Check sheet for the modelled part. Datum: model origin and axes. Units: mm. A direction names the side the tool comes from. Give positions to 0.01 mm unless a question says otherwise; leave off trailing zeros. Write each loop counter-clockwise with the first axis right and the second up, starting at its lowest first coordinate (ties: lowest second). Pieces come first, ordered by that corner, then holes. Notation, with made-up numbers: M 10,22 L 42,22 A21 cw 42,46 Z; hole C 69.25,-20.5 d10. An arc over 180 degrees is marked long. One line per item, written item: value. Start each with the question number.
from build123d import *

# Parameters (mm, degrees)
SKETCH1_W                 = 20.6
SKETCH1_H                 = 16
BOSS_EXTRUDE1_DEPTH       = 12.8
SKETCH2_W                 = 8.1
SKETCH2_H                 = 16
BOTTOM_CUT_DEPTH          = 1.1
FILL_PATTERN1_OUTLINE_W   = 8.1
FILL_PATTERN1_OUTLINE_H   = 16
FILL_PATTERN1_DEPTH       = 1.1
FILLET1_R                 = 2
SKETCH3_W                 = 8.1
SKETCH3_H                 = 14.8
TOP_CUT_DEPTH             = 7
M3X0_5_TAPPED_HOLE1_D     = 2.5
FILL_START                = 5.8
FILL_PATTERN2_OUTLINE_W   = 8.1
FILL_PATTERN2_OUTLINE_H   = 14.8
FILL_PATTERN2_DEPTH       = 7
FILL_START_2              = 1.1
FILL_PATTERN2_2_OUTLINE_R = 1.25
FILL_PATTERN2_2_DEPTH     = 4.7
SKETCH7_W                 = 1.5
SKETCH7_H                 = 4.4
BOSS_EXTRUDE2_DEPTH       = 4
CUT_EXTRUDE1_REACH        = 29.76
SKETCH8_R                 = 0.75
FILLET2_R                 = 0.5
LPATTERN1_COUNT           = 2
LPATTERN1_PITCH           = 10
FILLET2_OF_LPATTERN1_R    = 0.5
MIRROR1_START             = 8.8
MIRROR1_OUTLINE_R         = 0.75
MIRROR1_DEPTH             = 1.5


# Read off the part's stored shape, not the designer's step: Fill Pattern1, Fill Pattern2, Mirror1
with BuildPart() as part:
    # Sketch1 → Boss-Extrude1 (new body)
    with BuildSketch(Plane(origin=(0, 0, 0), x_dir=(1, 0, 0), z_dir=(0, 1, 0))):
        Rectangle(SKETCH1_W, SKETCH1_H)
    extrude(amount=BOSS_EXTRUDE1_DEPTH)

    # Sketch2 → BOTTOM CUT (cut)
    with BuildSketch(Plane.XZ):
        with Locations((-4.75, 0)):
            Rectangle(SKETCH2_W, SKETCH2_H)
    extrude(amount=-BOTTOM_CUT_DEPTH, mode=Mode.SUBTRACT)

    # Fill Pattern1 outline → Fill Pattern1 (cut)
    with BuildSketch(Plane(origin=(0, 0, 0), x_dir=(1, 0, 0), z_dir=(0, 1, 0))):
        with Locations((4.75, 0)):
            Rectangle(FILL_PATTERN1_OUTLINE_W, FILL_PATTERN1_OUTLINE_H)
    extrude(amount=FILL_PATTERN1_DEPTH, mode=Mode.SUBTRACT)

    # Fillet1
    fillet1_edges = [part.edges().sort_by_distance(p)[0] for p in [
        (0, 12.8, 8),
    ]]
    fillet(fillet1_edges, radius=FILLET1_R)

    # Sketch3 → TOP CUT (cut)
    with BuildSketch(Plane(origin=(0, 12.8, 0), x_dir=(1, 0, 0), z_dir=(0, 1, 0))):
        with Locations((-4.75, -0.6)):
            Rectangle(SKETCH3_W, SKETCH3_H)
    extrude(amount=-TOP_CUT_DEPTH, mode=Mode.SUBTRACT)

    # M3x0.5 Tapped Hole1 (through all)
    with Locations(Plane(origin=(0, 5.8, 0), x_dir=(1, 0, 0), z_dir=(0, 1, 0))):
        with Locations((-4.75, -1)):
            Hole(M3X0_5_TAPPED_HOLE1_D / 2)

    # Fill Pattern2 outline → Fill Pattern2 (cut)
    with BuildSketch(Plane(origin=(0, 0, 0), x_dir=(1, 0, 0), z_dir=(0, 1, 0)).offset(FILL_START)):
        with Locations((4.75, -0.6)):
            Rectangle(FILL_PATTERN2_OUTLINE_W, FILL_PATTERN2_OUTLINE_H)
    extrude(amount=FILL_PATTERN2_DEPTH, mode=Mode.SUBTRACT)

    # Fill Pattern2 2 outline → Fill Pattern2 2 (cut)
    with BuildSketch(Plane(origin=(0, 0, 0), x_dir=(1, 0, 0), z_dir=(0, 1, 0)).offset(FILL_START_2)):
        with Locations((4.75, -1)):
            Circle(FILL_PATTERN2_2_OUTLINE_R)
    extrude(amount=FILL_PATTERN2_2_DEPTH, mode=Mode.SUBTRACT)

    # Sketch7 → Boss-Extrude2 (add)
    with BuildSketch(Plane(origin=(0, 12.8, 0), x_dir=(1, 0, 0), z_dir=(0, 1, 0))):
        with Locations((-9.55, 5.8)):
            Rectangle(SKETCH7_W, SKETCH7_H)
    boss_extrude2 = extrude(amount=BOSS_EXTRUDE2_DEPTH)

    # Sketch8 → Cut-Extrude1 (cut, up to next)
    with BuildSketch(Plane.ZY.offset(10.3), mode=Mode.PRIVATE) as cut_extrude1_sk1:
        with Locations((-5.8, 14.8)):
            Circle(SKETCH8_R)
    cut_extrude1_tool1 = extrude(cut_extrude1_sk1.sketch, amount=-CUT_EXTRUDE1_REACH, mode=Mode.PRIVATE) & part.part
    cut_extrude1 = cut_extrude1_tool1.solids().sort_by_distance((-10.3, 14.8, -5.8))[0]
    add(cut_extrude1, mode=Mode.SUBTRACT)

    # Fillet2
    fillet2_edges = [part.edges().sort_by_distance(p)[0] for p in [
        (-9.55, 16.8, -3.6),
        (-9.55, 16.8, -8),
    ]]
    fillet(fillet2_edges, radius=FILLET2_R)

    # LPattern1: Boss-Extrude2, Cut-Extrude1 ×2
    with Locations(*[(0, 0, i * LPATTERN1_PITCH) for i in range(1, LPATTERN1_COUNT)]):
        add(boss_extrude2)
        add(cut_extrude1, mode=Mode.SUBTRACT)

    # Fillet2 of LPattern1
    fillet2_of_lpattern1_edges = [part.edges().sort_by_distance(p)[0] for p in [
        (-9.55, 16.8, 6.4),
        (-9.55, 16.8, 2),
    ]]
    fillet(fillet2_of_lpattern1_edges, radius=FILLET2_OF_LPATTERN1_R)

    # Mirror1 outline → Mirror1 (add)
    # profile 1 of 2: a face of its own
    with BuildSketch(Plane.YZ.offset(MIRROR1_START)):
        with BuildLine():
            ThreePointArc((16.8, -4.1), (16.653553391, -3.746446609), (16.3, -3.6))
            Line((16.3, -3.6), (12.8, -3.6))
            Line((12.8, -3.6), (12.8, -8))
            Line((12.8, -8), (16.3, -8))
            ThreePointArc((16.3, -8), (16.653553391, -7.853553391), (16.8, -7.5))
            Line((16.8, -7.5), (16.8, -4.1))
        make_face()
        with Locations((14.8, -5.8)):
            Circle(MIRROR1_OUTLINE_R, mode=Mode.SUBTRACT)
    # profile 2 of 2: a face of its own
    with BuildSketch(Plane.YZ.offset(MIRROR1_START)):
        with BuildLine():
            Line((12.8, 6.4), (12.8, 2))
            Line((12.8, 2), (16.3, 2))
            ThreePointArc((16.3, 2), (16.653553391, 2.146446609), (16.8, 2.5))
            Line((16.8, 2.5), (16.8, 5.9))
            ThreePointArc((16.8, 5.9), (16.653553391, 6.253553391), (16.3, 6.4))
            Line((16.3, 6.4), (12.8, 6.4))
        make_face()
        with Locations((14.8, 4.2)):
            Circle(MIRROR1_OUTLINE_R, mode=Mode.SUBTRACT)
    extrude(amount=MIRROR1_DEPTH)


solid = part.part
1) Cross-section at A-A (x = -4.75). Record the boundary of the cut face in (y, z).
2) Gauge pin test, flat ends, axial feed: pin 1 (6.5 mm diameter, centred on x = -4.5, z = 2.5, fed in from +Y); pin 2 (7 mm diameter, centred on x = 1, z = 2, fed in from +Y); pin 3 (0.8 mm diameter, centred on x = -10, y = 14.5, fed in from +Z). Record the tip position at first contact, or that the pin passes through.
3) Material ranges on L1, parallel to X at y = 11.5, z = 0; L2, parallel to Z at x = 4.75, y = 3.05; L3, parallel to Z at x = 9.9, y = 14.8, recorded low to high. Write a range as from..to.
4) Draft check along X on faces 1 (the flat face through (-8.8, 0.5, -0.1)), 2 (the flat face through (10, 12.8, -1)), 3 (the flat face through (-10.3, 8, 0)). Enter one of: released by +X, released by -X, zero draft, split by the parting line, or undercut.
5) Cross-section at B-B (y = 14.8). State how many separate pieces and enclosed holes the cut face has, plus the area to 3 significant figures.
6) Tool access check on faces 4 (the flat face through (8.8, 10, 0)), 5 (the flat face through (10, 15, -3.6)), 6 (the flat face through (0.7, 0.5, 0.1)), 7 (the flat face through (10, 15, 6.4)). Record the directions out of +Z, -Z, +X, -X, +Y, -Y that give a thin tool (end or side, any length) a straight path to the whole face; none if there is none.
7) Cross-section at D-D (y = 12.5). Record the boundary of the cut face in (x, z), plus the area to 3 significant figures.
8) Cross-section at C-C (z = 4.2). Record the boundary of the cut face in (x, y), plus the area to 3 significant figures.
Data:
1. outline: M 1.1,-8 L 12.8,-8 L 12.8,-6.8 L 5.8,-6.8 L 5.8,-0.25 L 1.1,-0.25 Z; M 1.1,2.25 L 5.8,2.25 L 5.8,8 L 1.1,8 Z
2. pin 1: stops at y = 5.8
2. pin 2: stops at y = 12.8
2. pin 3: stops at z = 6.4
3. L1: x = -10.3..-8.8, -0.7..0.7, 8.8..10.3
3. L2: z = -8..-0.25, 2.25..8
3. L3: z = -8..-6.55, -5.05..-3.6, 2..3.45, 4.95..6.4
4. face 1: undercut
4. face 2: zero draft
4. face 3: released by -X
5. separate pieces: 8
5. enclosed holes: 0
5. area: 17.4 mm2
6. face 4: +Z, +Y
6. face 5: +X, -X, +Y
6. face 6: +Z, -Z, -Y
6. face 7: +Z, +X, -X, +Y
7. outline: M -10.3,-8 L 10.3,-8 L 10.3,7.05 L 8.8,7.05 L 8.8,-6.8 L 0.7,-6.8 L 0.7,7.05 L -0.7,7.05 L -0.7,-6.8 L -8.8,-6.8 L -8.8,7.05 L -10.3,7.05 Z
7. area: 85.7 mm2
8. outline: M -10.3,0 L -8.8,0 L -8.8,1.1 L -0.7,1.1 L -0.7,0 L 0.7,0 L 0.7,1.1 L 8.8,1.1 L 8.8,0 L 10.3,0 L 10.3,14.05 L 8.8,14.05 L 8.8,5.8 L 0.7,5.8 L 0.7,12.8 L -0.7,12.8 L -0.7,5.8 L -8.8,5.8 L -8.8,14.05 L -10.3,14.05 Z; M -10.3,15.55 L -8.8,15.55 L -8.8,16.8 L -10.3,16.8 Z; M 8.8,15.55 L 10.3,15.55 L 10.3,16.8 L 8.8,16.8 Z
8. area: 140 mm2
